Could you check a few things on this model? Use its own coordinates, in mm. Face numbers are marked on the shaded views. A direction names the side the tool comes from. Give positions to 0.01 mm unless a question says otherwise; leave off trailing zeros. Order: outer loops, then holes, each group sorted by start corner. A loop starts at its lowest first (then second) coordinate and runs counter-clockwise, first axis right, second up. Notation, with made-up numbers: M -12.75,4.25 L -0.75,4.25 A38 cw -0.75,43.25 Z; hole C 68,-14.75 d11. An arc over 180 degrees is marked long. Use a Markdown table: item, result. Add a question column.
Item 1: If I drill on L1, parallel to X at y = 6, z = -0.5; L2, parallel to Y at x = -10, z = -15; L3, parallel to Z at x = -30.5, y = 0.75, over which ranges is the centre line in solid material (lowest first)? Write a range as from..to.
Item 2: For the marked faces 1, 2 and 3, which set-ups out of +Z, -Z, +X, -X, +Y, -Y let a thin tool reach every point of the face, with its end or its side?
Item 3: Suppose I cut it at B-B on x = 12.5. Write out the boundary of the cut face in (y, z), plus the area to 3 significant figures.
Item 4: Suppose I cut it at A-A on z = 0. Write out the boundary of the cut face in (x, y).
Item 5: Suppose I cut it at D-D on x = 46. Write out the boundary of the cut face in (y, z), plus the area to 3 significant figures.
Item 6: Suppose I cut it at C-C on y = 3.75. Write out the boundary of the cut face in (x, z).
Item 7: I'm going to push flat-ended pins straight in: pin 1 Ø1.8 at (y, z) = (0.5, -1) entering from -X; pin 2 Ø7 at (x, z) = (12.73, 12.73) entering from -Y; pin 3 Ø2 at (y, z) = (0.5, 18) entering from +X; pin 4 Ø5.5 at (x, z) = (-10, -12) entering from +Y. Where does each tip first touch, or does it pass through?
Item 8: If we mould it in two halves opening along X, with no side actions, what happens to the marked faces 4, 5 and 6? For each: released by +X, released by -X, zero draft, split by the parting line, or undercut.
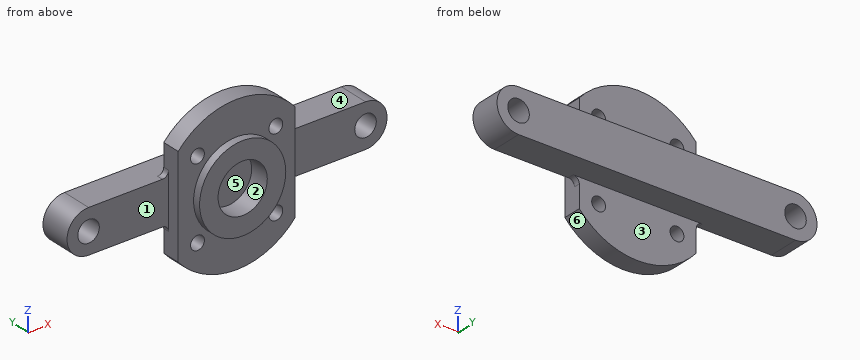
Autodesk Inventor part; units mm, degrees
ref_plane "Work Plane1" through (0, 2, 0) normal (0, 1, 0) x (-1, 0, 0)
ref_plane "YZ Plane" through (0, 0, 0) normal (1, 0, 0) x (0, 1, 0)
ref_plane "XY Plane" through (0, 0, 0) normal (0, 0, 1) x (1, 0, 0)
sketch "Sketch1" plane through (0, 0, 0) normal (0, 1, 0) x (-1, 0, 0)
  line L0 (0, 0) -> (45, 0) construction
  line L1 (0, 0) -> (52, 0)
  line L2 (0, 0) -> (-45, 0)
  line L3 (-45, 0) -> (45, 0) construction
  line L4 (-45, -7) -> (45, -7)
  line L5 (45, 7) -> (-45, 7)
  arc A0 (-45, 7) -> (-45, -7) centre (-45, 0) ccw
  arc A1 (45, -7) -> (45, 7) centre (45, 0) ccw
  circle A2 centre (45, 0) radius 3.5
  circle A3 centre (-45, 0) radius 3.5
  dimension "d0" = 45
  dimension "d1" = 52
  dimension "d2" = 45
  dimension "d3" = 7
extrude "Extrusion1" add sketch "Sketch1" along normal blind 10
ref_plane "Work Plane1" through (0, 2, 0) normal (0, 1, 0) x (-1, 0, 0)
sketch "Sketch2" plane through (0, 2, 0) normal (0, 1, 0) x (-1, 0, 0)
  line L0 (0, 0) -> (19, 0)
  line L1 (19, 0) -> (19, -16.2481)
  line L2 (19, 0) -> (19, 16.2481)
  line L3 (0, 0) -> (-19, 0)
  line L4 (-19, 0) -> (-19, -16.2481)
  line L5 (-19, 0) -> (-19, 16.2481)
  arc A0 (-19, -16.2481) -> (19, -16.2481) centre (0, 0) ccw
  arc A1 (19, 16.2481) -> (-19, 16.2481) centre (0, 0) ccw
  dimension "d8" = 19
  dimension "d10" = 19
extrude "Extrusion2" add sketch "Sketch2" against normal blind 6
fillet "Fillet1" radius 2 4 edges at (-19, 1, -7) (-19, 1, 7) (19, 1, -7) (19, 1, 7)
sketch "Sketch3" plane through (0, -4, 0) normal (0, -1, 0) x (1, 0, 0)
  circle A0 centre (0, 0) radius 18 construction
  line L0 (0, 0) -> (12.7279, 12.7279) construction
  line L1 (0, 0) -> (18, 0) construction
  circle A1 centre (12.7279, 12.7279) radius 2.25
  circle A2 centre (-12.7279, 12.7279) radius 2.25
  circle A3 centre (-12.7279, -12.7279) radius 2.25
  circle A4 centre (12.7279, -12.7279) radius 2.25
  dimension "d14" = 36
  dimension "d15" = 45
  dimension "d16" = 4.5
  dimension "d19" = 360
extrude "Extrusion3" cut sketch "Sketch3" against normal blind 10
sketch "Sketch4" plane through (0, -4, 0) normal (0, -1, 0) x (1, 0, 0)
  circle A0 centre (0, 0) radius 14
  circle A1 centre (0, 0) radius 8
  dimension "d23" = 28
  dimension "d24" = 16
extrude "Extrusion4" add sketch "Sketch4" along normal blind 2.5
sketch "Sketch5" plane through (0, -4, 0) normal (0, -1, 0) x (1, 0, 0)
  circle A0 centre (0, 0) radius 8
extrude "Extrusion5" cut sketch "Sketch5" against normal blind 4
properties part number "Coperchio inferiore"
Findings below:
| question | item | result |
|---|---|---|
| 1 | L1 | x = -51.98..-48.46, -41.54..41.54, 48.46..51.98 |
| 1 | L2 | y = -4..2 |
| 1 | L3 | z = -7..7 |
| 2 | face 1 | +Z, -Z, -X, -Y |
| 2 | face 2 | -Y |
| 2 | face 3 | -Z, +X, -X, +Y |
| 3 | outline | M -6.5,-6.3 L -4,-6.3 L -4,-10.49 L 2,-10.49 L 2,-7 L 10,-7 L 10,7 L 2,7 L 2,10.49 L -4,10.49 L -4,6.3 L -6.5,6.3 Z; M -4,-21.65 L 2,-21.65 L 2,-14.97 L -4,-14.97 Z; M -4,14.97 L 2,14.97 L 2,21.65 L -4,21.65 Z |
| 3 | area | 350 mm^2 |
| 4 | outline | M -52,0 L -48.5,0 L -48.5,10 L -52,10 Z; M -41.5,0 L -19,0 L -19,-4 L -14,-4 L -14,-6.5 L -8,-6.5 L -8,0 L 8,0 L 8,-6.5 L 14,-6.5 L 14,-4 L 19,-4 L 19,0 L 41.5,0 L 41.5,10 L -41.5,10 Z; M 48.5,0 L 52,0 L 52,10 L 48.5,10 Z |
| 5 | outline | M 0,-6.93 L 10,-6.93 L 10,-3.35 L 0,-3.35 Z; M 0,3.35 L 10,3.35 L 10,6.93 L 0,6.93 Z |
| 5 | area | 71.5 mm^2 |
| 6 | outline | M -45,-7 L 45,-7 A7 ccw 45,7 L -45,7 A7 ccw Z; hole C -45,0 d7; hole C 45,0 d7 |
| 7 | pin 1 | stops at x = -52 |
| 7 | pin 2 | stops at y = -4 |
| 7 | pin 3 | stops at x = 18.33 |
| 7 | pin 4 | stops at y = 2 |
| 8 | face 4 | zero draft |
| 8 | face 5 | undercut |
| 8 | face 6 | split by the parting line |
